For this review, take the finished solid that the model builds, in its own axes (mm). Round coordinates to 2 decimals unless told otherwise and drop trailing zeros. Order: outer loops, then holes, each group sorted by start corner. A loop starts at its lowest first (then second) coordinate and runs counter-clockwise, first axis right, second up. Notation, with made-up numbers: (50, 46) - (107, 46) arc R25 cw to (107, 62) - close; hole circle Ø4 at (18.5, 82.25). An arc over 180 degrees is marked (long way). One line per question, with ' | ' between items.
```python
from build123d import *

# Parameters (mm, degrees)
BOSS_EXTRUDE1_DEPTH = 1.5
SKETCH2_R           = 8
SKETCH2_R_2         = 6.75
CUT_EXTRUDE1_DEPTH  = 71.590509277


with BuildPart() as part:
    # Sketch1 → Boss-Extrude1 (new, symmetric)
    with BuildSketch(Plane(origin=(0, 0, 0), x_dir=(0, 0, -1), z_dir=(1, 0, 0))):
        with BuildLine():
            Line((-31, 31.9), (31, 31.9))
            ThreePointArc((31, 31.9), (62.9, 0), (31, -31.9))
            Line((31, -31.9), (-31, -31.9))
            ThreePointArc((-31, -31.9), (-62.9, 0), (-31, 31.9))
        make_face()
    extrude(amount=BOSS_EXTRUDE1_DEPTH, both=True)

    # Sketch2 → Cut-Extrude1 (cut, through all)
    with BuildSketch(Plane(origin=(1.5, 0, 0), x_dir=(0, 0, -1), z_dir=(1, 0, 0))):
        with Locations((-42.9, 0)):
            Circle(SKETCH2_R)
        with Locations((42.9, 0)):
            Circle(SKETCH2_R)
        with Locations((-14.3, 13.9)):
            Circle(SKETCH2_R_2)
        with Locations((14.3, 0)):
            Circle(SKETCH2_R)
        with Locations((-14.3, -13.9)):
            Circle(SKETCH2_R)
    extrude(amount=-CUT_EXTRUDE1_DEPTH, mode=Mode.SUBTRACT)


solid = part.part
```
(1) For probe 1 along Z at (x, y) = (0.45, 2); probe 2 along Z at (x, y) = (-0.8, -1.5); probe 3 along Y at (x, z) = (-0.15, -12.5), list the stretches that pass through material, from the lowest coordinate up. Write a range as [from, to].
Output values:
probe 1: [-62.84, -50.65], [-35.15, -22.05], [-6.55, 35.15], [50.65, 62.84] | probe 2: [-62.86, -50.76], [-35.04, -22.16], [-6.44, 35.04], [50.76, 62.86] | probe 3: [-31.9, -7.79], [7.79, 31.9]
(2) We need section B-B on y = -19. State the section outline as (x, z) points, plus the area to 3 significant figures.
Output values:
outline: (-1.5, -56.62) - (1.5, -56.62) - (1.5, 8.14) - (-1.5, 8.14) - close; (-1.5, 20.46) - (1.5, 20.46) - (1.5, 56.62) - (-1.5, 56.62) - close | area: 303 mm^2
(3) We need section C-C on x = 0.6. State the section outline as (y, z) points.
Output values:
outline: (-31.9, -31) arc R31.9 ccw to (31.9, -31) - (31.9, 31) arc R31.9 ccw to (-31.9, 31) - close; hole circle Ø16 at (-13.9, 14.3); hole circle Ø16 at (0, -42.9); hole circle Ø16 at (0, -14.3); hole circle Ø16 at (0, 42.9); hole circle Ø13.5 at (13.9, 14.3)
(4) We need section D-D on z = 14.3. State the section outline as (x, y) points, plus the area to 3 significant figures.
Output values:
outline: (-1.5, -31.9) - (1.5, -31.9) - (1.5, -21.9) - (-1.5, -21.9) - close; (-1.5, -5.9) - (1.5, -5.9) - (1.5, 7.15) - (-1.5, 7.15) - close; (-1.5, 20.65) - (1.5, 20.65) - (1.5, 31.9) - (-1.5, 31.9) - close | area: 103 mm^2
(5) Mouldability with a two-part tool opening along Z and no side actions: class faces 1 (the cylindrical face through (0.021, 0.701, -62.892)), 2 (the flat face through (0, 31.9, 0)), 3 (the cylindrical face through (0.021, -0.701, 62.892)), 4 (the cylindrical face through (0.02, -7.1, -17.99)) as released by +Z, released by -Z, zero draft, split by the parting line, or undercut.
Output values:
face 1: released by -Z | face 2: zero draft | face 3: released by +Z | face 4: undercut
(6) We need section A-A on z = -14.3. State the section outline as (x, y) points.
Output values:
outline: (-1.5, -31.9) - (1.5, -31.9) - (1.5, -8) - (-1.5, -8) - close; (-1.5, 8) - (1.5, 8) - (1.5, 31.9) - (-1.5, 31.9) - close
